```python
from build123d import *

# Parameters (mm, degrees)
SKETCH_2_R      = 3.85
SKETCH_2_R_2    = 1.65
EXTRUDE_8_DEPTH = 3.35
SKETCH_3_R      = 5.2
EXTRUDE_9_DEPTH = 2


with BuildPart() as part:
    # 草图2 → 凸台-拉伸8 (new body)
    with BuildSketch(Plane(origin=(0, 0, 0), x_dir=(1, 0, 0), z_dir=(0, 1, 0))):
        with Locations(Location((0, 0, 0), (0, 0, 270))):
            Circle(SKETCH_2_R)
        with Locations(Location((0, 0, 0), (0, 0, 270))):
            Circle(SKETCH_2_R_2, mode=Mode.SUBTRACT)
    extrude(amount=-EXTRUDE_8_DEPTH)

    # 草图3 → 凸台-拉伸9 (add)
    with BuildSketch(Plane(origin=(0, -3.35, 0), x_dir=(-1, 0, 0), z_dir=(0, -1, 0))):
        with Locations(Location((0, 0, 0), (0, 0, 90))):
            Circle(SKETCH_3_R)
    extrude(amount=EXTRUDE_9_DEPTH)

    # 切除-放样1: read off the stored shape, not the designer's step
    # 切除-放样1: loft between two sections, ruled curve by curve
    loft_1_from = [
        Edge.make_bspline([(0.764858596, -5.35, -3.56896222), (-6.373065844, -5.35, -5.098679412), (-7.902783036, -5.35, 2.039245028), (-0.764858596, -5.35, 3.56896222), (6.373065844, -5.35, 5.098679412), (7.902783036, -5.35, -2.039245028), (0.764858596, -5.35, -3.56896222)], [0, 0, 0, 0, 0.5, 0.5, 0.5, 1, 1, 1, 1], 3, [1, 0.333333333, 0.333333333, 1, 0.333333333, 0.333333333, 1]),
    ]
    loft_1_to = [
        Edge.make_bspline([(-0.535444465, -3.35, -1.56070472), (-3.656853906, -3.35, -0.48981579), (-2.585964976, -3.35, 2.631593651), (0.535444465, -3.35, 1.56070472), (3.656853906, -3.35, 0.48981579), (2.585964976, -3.35, -2.631593651), (-0.535444465, -3.35, -1.56070472)], [0, 0, 0, 0, 0.5, 0.5, 0.5, 1, 1, 1, 1], 3, [1, 0.333333333, 0.333333333, 1, 0.333333333, 0.333333333, 1]),
    ]
    loft_1 = Solid(Shell([*[Face.make_surface_from_curves(loft_1_from[k], loft_1_to[k]) for k in range(1)], Face(Wire(loft_1_from)), Face(Wire(loft_1_to))]))
    add(loft_1, mode=Mode.SUBTRACT)


solid = part.part
```
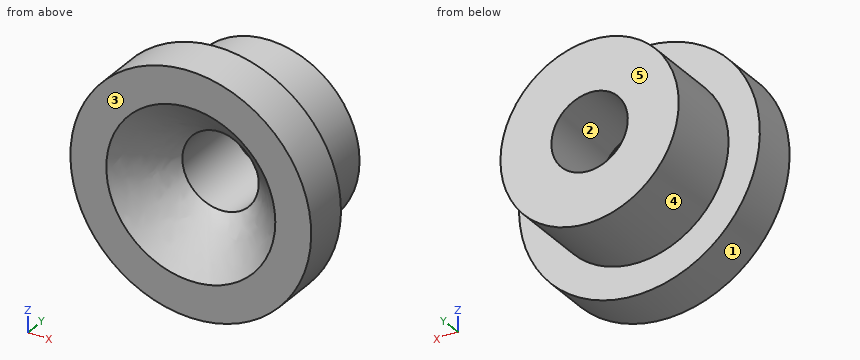
The model under review builds one solid part; all positions refer to its coordinate system, in mm. Face numbers are marked on the shaded views. A direction names the side the tool comes from. Round coordinates to 2 decimals unless told otherwise and drop trailing zeros. Loops run counter-clockwise (first coordinate to the right, second up) from the corner with the lowest first, then second, coordinate; pieces in that order, holes last.
Item 1: Mouldability with a two-part tool opening along Z and no side actions: class the marked faces 1, 2 and 3 as released by +Z, released by -Z, zero draft, split by the parting line, or undercut.
Determined:
face 1: split by the parting line
face 2: undercut
face 3: zero draft
Item 2: For the marked faces 4 and 5, list the 3-axis set-ups (+Z, -Z, +X, -X, +Y, -Y) from which the entire face can be reached by the end or side of a thin tool; tool diameter is ignored.
Determined:
face 4: +Y
face 5: +Z, -Z, +X, -X, +Y
Item 3: Clearance check with flat-ended pins moving along their axes: pin 1 Ø3 at (x, y) = (0, -2) entering from +Z; pin 2 Ø1.5 at (y, z) = (-4.5, -4) entering from -X. State where each tip first meets the part, or that it passes through.
Determined:
pin 1: stops at z = 5.2
pin 2: stops at x = -4.06
Item 4: For line 1 (X direction, y = -1.2, z = 0); line 2 (Y direction, x = -3, z = 3.25), list the stretches that pass through material, from the lowest coordinate up.
Determined:
line 1: x = -3.85 to -1.65, 1.65 to 3.85
line 2: y = -5.35 to -3.35
Item 5: Take a section at A-A (y = -2.8). Write out the cut boundary in (x, z).
Determined:
outline: circle Ø7.7 at (0, 0); hole circle Ø3.3 at (0, 0)
Item 6: Take a section at C-C (z = 4.75). Write out the cut boundary in (x, y), then the cut area to 3 significant figures.
Determined:
outline: (-2.12, -5.35) - (2.12, -5.35) - (2.12, -3.35) - (-2.12, -3.35) - close
area: 8.46 mm2
Item 7: Take a section at B-B (x = -4). Write out the cut boundary in (y, z), then the cut area to 3 significant figures.
Determined:
outline: (-5.35, -3.32) - (-3.35, -3.32) - (-3.35, 3.32) - (-5.35, 3.32) - close
area: 13.3 mm2
